Input: dimensioned drawing with shaded views. Units: mm. Origin: part minimum x, y, z. A direction names the side the tool comes from. Give positions to 0.01 mm unless a question says otherwise; leave off trailing zeros. Write each loop counter-clockwise with the first axis right and the second up, starting at its lowest first coordinate (ties: lowest second). Pieces come first, ordered by that corner, then holes. Notation, with made-up numbers: (40, 20) -> (96, 20) arc R27 cw to (96, 54) -> close; hole circle Ø5 at (25, 41). An arc over 180 degrees is marked (long way). Answer as a JSON object with one key per item and string values. Group by question number.
(1) Contact query for flat-ended pins moving along their axis: pin 1 Ø1.2 at (x, z) = (12.5, 1) entering from -Y; pin 2 Ø1.2 at (y, z) = (56, 1.5) entering from -X; pin 3 Ø0.5 at (x, z) = (15.5, 2) entering from +Y. Output: stop coordinate, or through.
(2) Material intervals for probe 1 along Y at (x, z) = (25, 1.95); probe 2 along Y at (x, z) = (4, 1.35); probe 3 along X at (y, z) = (42, 1.85), sorted ascending.
(3) Section query C-C on x = 25. Output: boundary loops of the cut face in (y, z).
(4) Section query A-A on y = 55. Output: boundary loops of the cut face in (x, z).
(5) Set-up query: the marked faces 1 and 2. Return all of +Z, -Z, +X, -X, +Y, -Y with unobstructed straight access to the full face (end or side cutting, diameter ignored); none if empty.
(6) Section query B-B on z = 1.35. Output: boundary loops of the cut face in (x, y), plus the area to 3 significant figures.
(7) Draft query along Y for the marked faces 3 and 4. Return one class per face: +Y half, -Y half, draft (parallel to the pull), parting line (faces both ways), or undercut.
(8) Section query D-D on x = 14.5. Output: boundary loops of the cut face in (y, z).
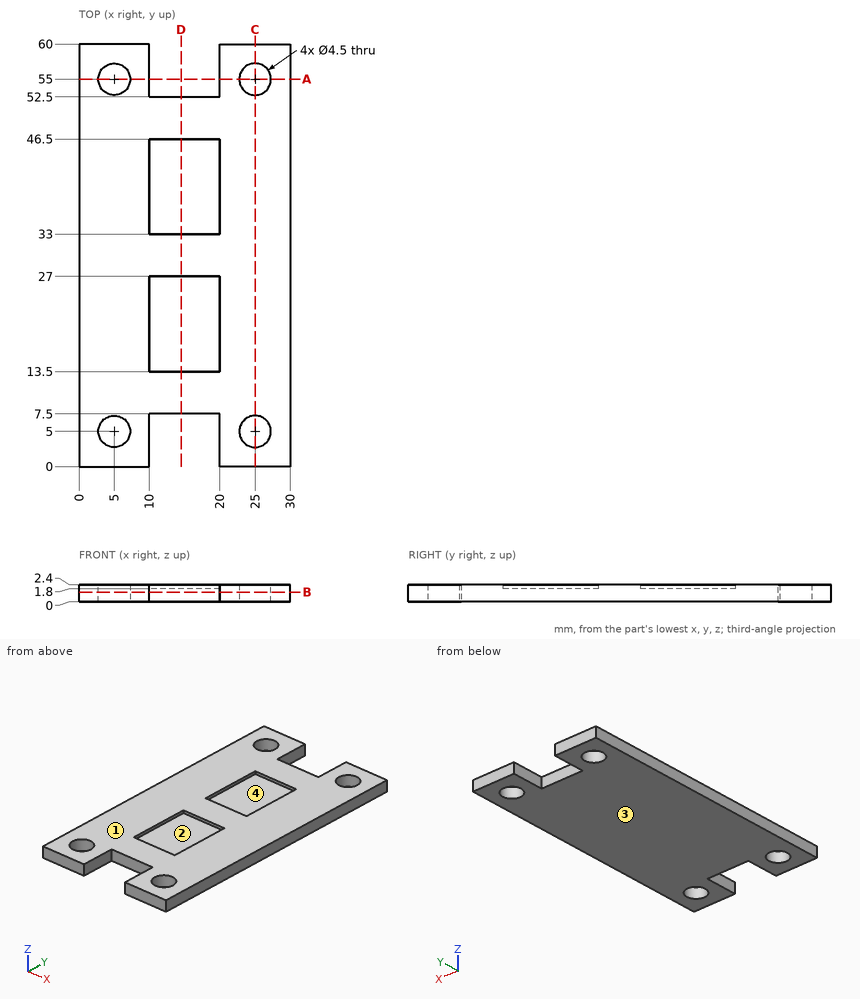
Answer list:
{
 "1": {"pin 1": "y = 7.5", "pin 2": "x = 0", "pin 3": "y = 52.5"},
 "2": {"probe 1": "0 to 2.75, 7.25 to 52.75, 57.25 to 60", "probe 2": "0 to 2.98, 7.02 to 52.98, 57.02 to 60", "probe 3": "0 to 10, 20 to 30"},
 "3": {"outline": "(0, 0) -> (2.75, 0) -> (2.75, 2.4) -> (0, 2.4) -> close; (7.25, 0) -> (52.75, 0) -> (52.75, 2.4) -> (7.25, 2.4) -> close; (57.25, 0) -> (60, 0) -> (60, 2.4) -> (57.25, 2.4) -> close"},
 "4": {"outline": "(0, 0) -> (2.75, 0) -> (2.75, 2.4) -> (0, 2.4) -> close; (7.25, 0) -> (10, 0) -> (10, 2.4) -> (7.25, 2.4) -> close; (20, 0) -> (22.75, 0) -> (22.75, 2.4) -> (20, 2.4) -> close; (27.25, 0) -> (30, 0) -> (30, 2.4) -> (27.25, 2.4) -> close"},
 "5": {"face 1": "+Z, +X, -X, +Y, -Y", "face 2": "+Z"},
 "6": {"outline": "(0, 0) -> (10, 0) -> (10, 7.5) -> (20, 7.5) -> (20, 0) -> (30, 0) -> (30, 60) -> (20, 60) -> (20, 52.5) -> (10, 52.5) -> (10, 60) -> (0, 60) -> close; hole circle Ø4.5 at (5, 5); hole circle Ø4.5 at (5, 55); hole circle Ø4.5 at (25, 5); hole circle Ø4.5 at (25, 55)", "area": "1,590 mm2"},
 "7": {"face 3": "draft", "face 4": "undercut"},
 "8": {"outline": "(7.5, 0) -> (52.5, 0) -> (52.5, 2.4) -> (46.5, 2.4) -> (46.5, 1.8) -> (33, 1.8) -> (33, 2.4) -> (27, 2.4) -> (27, 1.8) -> (13.5, 1.8) -> (13.5, 2.4) -> (7.5, 2.4) -> close"}
}
